from build123d import *

# Parameters (mm, degrees)
F0_W     = 30
F0_H     = 4
F1_DEPTH = 3


with BuildPart() as f1:
    # F0 (on Front) → F1 (new body)
    with BuildSketch(Plane.XZ):
        Polygon((33, 10), (-33, 10), (-33, 6), (-30, 6), (-30, -6), (-33, -6), (-33, -10), (33, -10), (33, -6), (30, -6), (30, 6), (33, 6), align=None)
        Rectangle(F0_W, F0_H, mode=Mode.SUBTRACT)
    extrude(amount=F1_DEPTH)


solid = f1.part
Input: part model. Units: mm. Frame: model coordinates. A direction names the side the tool comes from. Give positions to 0.01 mm unless a question says otherwise; leave off trailing zeros. Loops run counter-clockwise (first coordinate to the right, second up) from the corner with the lowest first, then second, coordinate; pieces in that order, holes last. Notation, with made-up numbers: M 68.25,-8 L 120.25,-8 A13 cw 120.25,-2 Z; hole C 79,73.25 d8. An arc over 180 degrees is marked long. Use CSV: the item, a comma, the result in double quotes.
(1) Section A-A, the plane z = 0.5. Return loops of the section in (x, y).
Outcome:
outline,"M -30,-3 L -15,-3 L -15,0 L -30,0 Z; M 15,-3 L 30,-3 L 30,0 L 15,0 Z"
(2) Section D-D, the plane z = 4. Return loops of the section in (x, y).
Outcome:
outline,"M -30,-3 L 30,-3 L 30,0 L -30,0 Z"
(3) Section C-C, the plane y = -0.65. Return loops of the section in (x, z), plus the area to 3 significant figures.
Outcome:
outline,"M -33,-10 L 33,-10 L 33,-6 L 30,-6 L 30,6 L 33,6 L 33,10 L -33,10 L -33,6 L -30,6 L -30,-6 L -33,-6 Z; hole M -15,-2 L 15,-2 L 15,2 L -15,2 Z"
area,"1,130 mm²"
(4) Pin query (flat end, axial travel): P1, Ø0.9, axis at y = -1, z = -3, coming from the -X side; P2, Ø1.5, axis at y = -2, z = 0, coming from the +X side. Return the tip coordinate at first contact, or that it passes through.
Outcome:
P1,"stops at x = -30"
P2,"stops at x = 30"
(5) Set-up query: faces 1 (the face through (32, -1, -6)), 2 (the face through (0, -1, 2)), 3 (the face through (-32, -1, 6)), 4 (the face through (-0.5, 0, 2.4)). Return all of +Z, -Z, +X, -X, +Y, -Y with unobstructed straight access to the full face (end or side cutting, diameter ignored); none if empty.
Outcome:
face 1,"+X, +Y, -Y"
face 2,"+Y, -Y"
face 3,"-X, +Y, -Y"
face 4,"+Z, -Z, +X, -X, +Y"
(6) Material intervals for L1, parallel to X at y = -1.05, z = -1.75; L2, parallel to Z at x = -8.5, y = -0.4; L3, parallel to X at y = -1.4, z = -4, sorted ascending. Write a range as [from, to].
Outcome:
L1,"x = [-30, -15], [15, 30]"
L2,"z = [-10, -2], [2, 10]"
L3,"x = [-30, 30]"
(7) Section B-B, the plane x = -3.5. Return loops of the section in (y, z), plus the area to 3 significant figures.
Outcome:
outline,"M -3,-10 L 0,-10 L 0,-2 L -3,-2 Z; M -3,2 L 0,2 L 0,10 L -3,10 Z"
area,"48.0 mm²"
(8) Pull-direction query (Z, two-part tool) for faces 5 (the face through (15, -1, 0)), 6 (the face through (33, -1, -8)), 7 (the face through (0, -1, 10)); classes: pulls with the +Z half, pulls with the -Z half, needs draft (parallel to the pull), parting line crosses it, or undercut.
Outcome:
face 5,"undercut"
face 6,"needs draft"
face 7,"pulls with the +Z half"
